Work out the finished part from the listing and answer in its coordinate system (mm). Round coordinates to 2 decimals unless told otherwise and drop trailing zeros. Order: outer loops, then holes, each group sorted by start corner. A loop starts at its lowest first (then second) coordinate and runs counter-clockwise, first axis right, second up. Notation, with made-up numbers: (79, 73.5) -> (106, 73.5) arc R24 ccw to (106, 108.5) -> close; hole circle Ø4 at (64.25, 53). An arc over 180 degrees is marked (long way). Use one line per item in the form item = value.
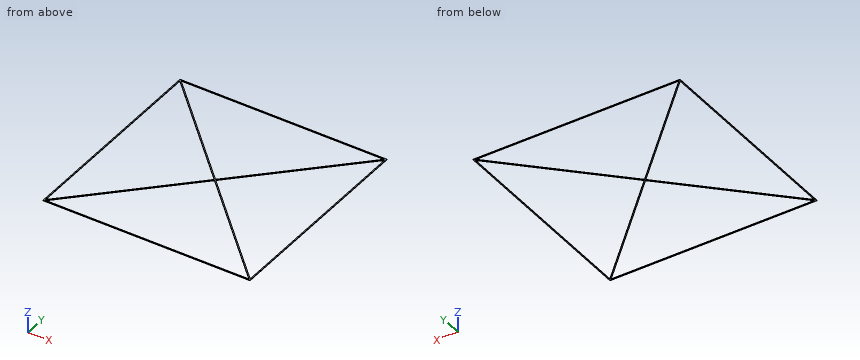
```python
from build123d import *

# Parameters (mm, degrees)
F2_DEPTH = 0.21


with BuildPart() as f2:
    # F1 (on Top) → F2 (new body)
    with BuildSketch(Plane.XY):
        Polygon((-40, 40), (-40, 0), (-39.59, 0), (-39.59, 39.3000862197), (-39.59, 39.59), (-39.3000862197, 39.59), (0, 39.59), (0, 40), align=None)
        Polygon((-40, -40), (40, -40), (40, 40), (0, 40), (0, 39.59), (39.3000862197, 39.59), (39.59, 39.59), (39.59, 39.3000862197), (39.59, -39.3000862197), (39.59, -39.59), (39.3000862197, -39.59), (-39.3000862197, -39.59), (-39.59, -39.59), (-39.59, -39.3000862197), (-39.59, 0), (-40, 0), align=None)
        Polygon((-39.59, 39.59), (-39.59, 39.3000862197), (-0.2899137803, 0), (-0.1449568901, 0.1449568901), align=None)
        Polygon((0, 0.2899137803), (-39.3000862197, 39.59), (-39.59, 39.59), (-0.1449568901, 0.1449568901), align=None)
        Polygon((39.59, 39.59), (39.3000862197, 39.59), (0, 0.2899137803), (0.1449568901, 0.1449568901), align=None)
        Polygon((39.59, 39.3000862197), (39.59, 39.59), (0.1449568901, 0.1449568901), (0.2899137803, 0), align=None)
        Polygon((0.2899137803, 0), (0.1449568901, 0.1449568901), (0, 0), (0.1449568901, -0.1449568901), align=None)
        Polygon((0.1449568901, 0.1449568901), (0, 0.2899137803), (-0.1449568901, 0.1449568901), (0, 0), align=None)
        Polygon((-0.1449568901, 0.1449568901), (-0.2899137803, 0), (-0.1449568901, -0.1449568901), (0, 0), align=None)
        Polygon((0, 0), (-0.1449568901, -0.1449568901), (0, -0.2899137803), (0.1449568901, -0.1449568901), align=None)
        Polygon((0, -0.2899137803), (39.3000862197, -39.59), (39.59, -39.59), (0.1449568901, -0.1449568901), align=None)
        Polygon((39.59, -39.59), (39.59, -39.3000862197), (0.2899137803, 0), (0.1449568901, -0.1449568901), align=None)
        Polygon((-0.1449568901, -0.1449568901), (-39.59, -39.59), (-39.3000862197, -39.59), (0, -0.2899137803), align=None)
        Polygon((-0.2899137803, 0), (-39.59, -39.3000862197), (-39.59, -39.59), (-0.1449568901, -0.1449568901), align=None)
    extrude(amount=F2_DEPTH)


solid = f2.part
```
Item 1: Consider line 1 along X through (y, z) = (8, 0.05); line 2 along X through (y, z) = (-31.5, 0.1); line 3 along Y through (x, z) = (-7, 0.1). Determine where each line is inside the solid, lowest interval first.
Findings:
line_1 = -40 to -39.59, -8.29 to -7.71, 7.71 to 8.29, 39.59 to 40
line_2 = -40 to -39.59, -31.79 to -31.21, 31.21 to 31.79, 39.59 to 40
line_3 = -40 to -39.59, -7.29 to -6.71, 6.71 to 7.29, 39.59 to 40
Item 2: The part is cut by section C-C, the plane x = -7. Give the vertices of the cut face in (y, z).
Findings:
outline = (-40, 0) -> (-39.59, 0) -> (-39.59, 0.21) -> (-40, 0.21) -> close; (-7.29, 0) -> (-6.71, 0) -> (-6.71, 0.21) -> (-7.29, 0.21) -> close; (6.71, 0) -> (7.29, 0) -> (7.29, 0.21) -> (6.71, 0.21) -> close; (39.59, 0) -> (40, 0) -> (40, 0.21) -> (39.59, 0.21) -> close
Item 3: The part is cut by section A-A, the plane z = 0.15. Give the vertices of the cut face in (x, y), and give its area (3 significant figures).
Findings:
outline = (-40, -40) -> (40, -40) -> (40, 40) -> (-40, 40) -> close; hole (-39.59, -39.3) -> (-0.29, 0) -> (-39.59, 39.3) -> close; hole (-39.3, -39.59) -> (39.3, -39.59) -> (0, -0.29) -> close; hole (-39.3, 39.59) -> (0, 0.29) -> (39.3, 39.59) -> close; hole (0.29, 0) -> (39.59, -39.3) -> (39.59, 39.3) -> close
area = 222 mm^2
Item 4: The part is cut by section B-B, the plane y = -22. Give the vertices of the cut face in (x, z).
Findings:
outline = (-40, 0) -> (-39.59, 0) -> (-39.59, 0.21) -> (-40, 0.21) -> close; (-22.29, 0) -> (-21.71, 0) -> (-21.71, 0.21) -> (-22.29, 0.21) -> close; (21.71, 0) -> (22.29, 0) -> (22.29, 0.21) -> (21.71, 0.21) -> close; (39.59, 0) -> (40, 0) -> (40, 0.21) -> (39.59, 0.21) -> close
